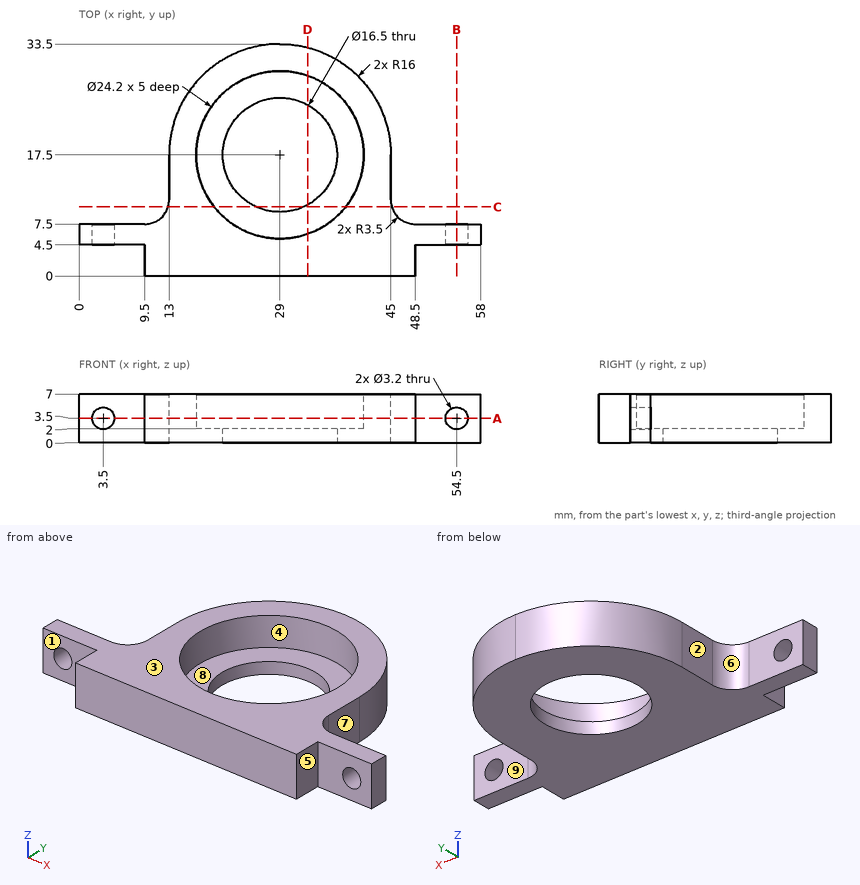
Study the drawing (mm; zero at the part's minimum x, y, z) and answer. A direction names the side the tool comes from. Coordinates: 2 decimals unless noted, no trailing zeros. Loops run counter-clockwise (first coordinate to the right, second up) from the corner with the lowest first, then second, coordinate; pieces in that order, holes last. Notation, with made-up numbers: (78.5, -9.75) -> (125.5, -9.75) arc R18 cw to (125.5, 10.25) -> close; hole circle Ø10 at (-23, 83.5). An arc over 180 degrees is marked (long way). Answer in a Markdown table with one row per item. Add a question column.
1. The part is cut by section B-B, the plane x = 54.5. Write down the section's boundary in (y, z).
2. Determine the mould class of the marked faces 6, 7, 8 and 9 for opening direction X: +X half, -X half, draft (parallel to the pull), parting line (faces both ways), or undercut.
3. For the marked faces 1, 2, 3, 4 and 5, determine the directions among +Z, -Z, +X, -X, +Y, -Y from which every point of the face is accessible in a straight line to the end or side of a thin tool.
4. The part is cut by section C-C, the plane y = 10. Write down the section's boundary in (x, z), then the cut area to 3 significant figures.
5. The part is cut by section A-A, the plane z = 3.5. Count the separate pieces of the cut face and the enclosed holes in it, then the cut area to 3 significant figures.
6. Flat-ended cylindrical pins translate along their axes: P1, Ø3.5, axis at y = 14.5, z = 4, coming from the -X side; P2, Ø3.5, axis at x = 52, z = 2, coming from the -Y side; P3, Ø2, axis at x = 2.5, z = 3, coming from the +Y side. Find the tip coordinate at first contact, or state that the pin passes through.
7. The part is cut by section D-D, the plane x = 33. Write down the section's boundary in (y, z), then the cut area to 3 significant figures.
8. Consider line 1 (X direction, y = 5.1, z = 3.5); line 2 (X direction, y = 17.5, z = 5); line 3 (X direction, y = 6.3, z = 3.5). Determine where each line is inside the solid, lowest interval first. Write a range as [from, to].
Answer below:
| question | item | result |
|---|---|---|
| 1 | outline | (4.5, 0) -> (7.5, 0) -> (7.5, 1.9) -> (4.5, 1.9) -> close; (4.5, 5.1) -> (7.5, 5.1) -> (7.5, 7) -> (4.5, 7) -> close |
| 2 | face 6 | -X half |
| 2 | face 7 | +X half |
| 2 | face 8 | undercut |
| 2 | face 9 | draft |
| 3 | face 1 | +Z, -Z, -X, -Y |
| 3 | face 2 | +Z, -Z, -X, +Y |
| 3 | face 3 | +Z, +X, -X, +Y, -Y |
| 3 | face 4 | +Z |
| 3 | face 5 | +Z, -Z, +X, -Y |
| 4 | outline | (12.85, 0) -> (25.56, 0) -> (25.56, 2) -> (19.5, 2) -> (19.5, 7) -> (12.85, 7) -> close; (32.44, 0) -> (45.15, 0) -> (45.15, 7) -> (38.5, 7) -> (38.5, 2) -> (32.44, 2) -> close |
| 4 | area | 117 mm2 |
| 5 | separate pieces | 3 |
| 5 | enclosed holes | 1 |
| 5 | area | 598 mm2 |
| 6 | P1 | x = 13 |
| 6 | P2 | y = 4.5 |
| 6 | P3 | y = 7.5 |
| 7 | outline | (0, 0) -> (10.28, 0) -> (10.28, 2) -> (6.08, 2) -> (6.08, 7) -> (0, 7) -> close; (24.72, 0) -> (32.99, 0) -> (32.99, 7) -> (28.92, 7) -> (28.92, 2) -> (24.72, 2) -> close |
| 7 | area | 87.9 mm2 |
| 8 | line 1 | [0, 1.9], [5.1, 52.9], [56.1, 58] |
| 8 | line 2 | [13, 16.9], [41.1, 45] |
| 8 | line 3 | [0, 1.9], [5.1, 24.42], [33.58, 52.9], [56.1, 58] |
